Geometry: final body of the model. Coordinates: model frame, mm. Give positions to 0.01 mm unless a question says otherwise; leave off trailing zeros. Loops run counter-clockwise (first coordinate to the right, second up) from the corner with the lowest first, then second, coordinate; pieces in that order, holes last.
from build123d import *

# Parameters (mm, degrees)
F0_R           = 3.3999999346
F0_R_2         = 4.4999999135
F1_DEPTH       = 15
F2_D           = 8.8
F2_CBORE_D     = 15
F2_CBORE_DEPTH = 8
F3_D           = 8.8
F3_CBORE_D     = 15
F3_CBORE_DEPTH = 8.6
F4_D           = 8.8
F5_D           = 7.2


with BuildPart() as f1:
    # F0 (on Front) → F1 (new body)
    with BuildSketch(Plane.XZ):
        Polygon((25.9961503957, 121.2465122815), (-26.0038496043, 121.2465122815), (-34.0038514504, 113.2465114353), (-34.0038514504, -70.7534860262), (-26.0038496043, -78.7534868724), (25.9961503957, -78.7534868724), (33.9961512419, -70.7534860262), (33.9961512419, 113.2465114353), align=None)
        with Locations((-23.2538496572, -28.7534868339)):
            Circle(F0_R, mode=Mode.SUBTRACT)
        with Locations((-0.0038501043, -63.7534861608)):
            Circle(F0_R_2, mode=Mode.SUBTRACT)
        with Locations((23.2461494486, -28.7534868339)):
            Circle(F0_R, mode=Mode.SUBTRACT)
        with Locations((-23.2538496572, 71.246511243)):
            Circle(F0_R, mode=Mode.SUBTRACT)
        with Locations((23.2461494486, 71.246511243)):
            Circle(F0_R, mode=Mode.SUBTRACT)
        with Locations((-0.0038501043, 106.2465105699)):
            Circle(F0_R_2, mode=Mode.SUBTRACT)
    extrude(amount=F1_DEPTH)

    # F2 (through all)
    with Locations(Plane(origin=(0, 0, 0), x_dir=(1, 0, 0), z_dir=(0, 1, 0))):
        with Locations((-0.0038501043, -106.2465105699)):
            CounterBoreHole(F2_D / 2, F2_CBORE_D / 2, F2_CBORE_DEPTH)

    # F3 (through all)
    with Locations(Plane(origin=(0, 0, 0), x_dir=(1, 0, 0), z_dir=(0, 1, 0))):
        with Locations((-0.0038501043, 63.7534861608)):
            CounterBoreHole(F3_D / 2, F3_CBORE_D / 2, F3_CBORE_DEPTH)

    # F4 (through all)
    with Locations(Plane(origin=(0, 0, 0), x_dir=(1, 0, 0), z_dir=(0, 1, 0))):
        with Locations((23.2461494486, 28.7534868339)):
            Hole(F4_D / 2)

    # F5 (through all)
    with Locations(Plane(origin=(0, 0, 0), x_dir=(1, 0, 0), z_dir=(0, 1, 0))):
        with Locations((0, 0)):
            Hole(F5_D / 2)


solid = f1.part
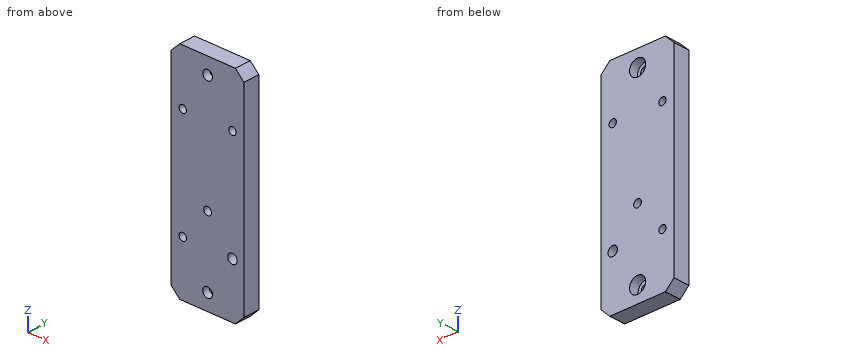
Item 1: Section query A-A on z = 0. Return loops of the section in (x, y), plus the area to 3 significant figures.
Values follow:
outline: (-34, -15) - (-3.6, -15) - (-3.6, 0) - (-34, 0) - close; (3.6, -15) - (34, -15) - (34, 0) - (3.6, 0) - close
area: 912 mm2
Item 2: Section query B-B on x = 0. Return loops of the section in (y, z).
Values follow:
outline: (-15, -78.75) - (0, -78.75) - (0, -71.25) - (-8.6, -71.25) - (-8.6, -68.25) - (-15, -68.25) - close; (-15, -59.25) - (-8.6, -59.25) - (-8.6, -56.25) - (0, -56.25) - (0, -3.6) - (-15, -3.6) - close; (-15, 3.6) - (0, 3.6) - (0, 98.75) - (-8, 98.75) - (-8, 101.75) - (-15, 101.75) - close; (-15, 110.75) - (-8, 110.75) - (-8, 113.75) - (0, 113.75) - (0, 121.25) - (-15, 121.25) - close
Item 3: Section query D-D on y = -4.25. Return loops of the section in (x, z).
Values follow:
outline: (-34, -70.75) - (-26, -78.75) - (26, -78.75) - (34, -70.75) - (34, 113.25) - (26, 121.25) - (-26, 121.25) - (-34, 113.25) - close; hole circle Ø6.8 at (-23.25, -28.75); hole circle Ø6.8 at (-23.25, 71.25); hole circle Ø15 at (0, -63.75); hole circle Ø15 at (0, 106.25); hole circle Ø7.2 at (0, 0); hole circle Ø8.8 at (23.25, -28.75); hole circle Ø6.8 at (23.25, 71.25)
Item 4: Ray query, probe 1 along Z at (x, y) = (0, -8.5); probe 2 along Z at (x, y) = (3, -4.5); probe 3 along Z at (x, y) = (22, -7.25). Return the intervals inside material, ascending.
Values follow:
probe 1: z = -78.75 to -71.25, -56.25 to -3.6, 3.6 to 101.75, 110.75 to 121.25
probe 2: z = -78.75 to -70.63, -56.88 to -1.99, 1.99 to 99.37, 113.12 to 121.25
probe 3: z = -78.75 to -32.97, -24.53 to 68.08, 74.41 to 121.25
Item 5: Section query C-C on y = -12.5. Return loops of the section in (x, z).
Values follow:
outline: (-34, -70.75) - (-26, -78.75) - (26, -78.75) - (34, -70.75) - (34, 113.25) - (26, 121.25) - (-26, 121.25) - (-34, 113.25) - close; hole circle Ø6.8 at (-23.25, -28.75); hole circle Ø6.8 at (-23.25, 71.25); hole circle Ø9 at (0, -63.75); hole circle Ø9 at (0, 106.25); hole circle Ø7.2 at (0, 0); hole circle Ø8.8 at (23.25, -28.75); hole circle Ø6.8 at (23.25, 71.25)
Item 6: Pin query (flat end, axial travel): pin 1 (8 mm diameter, centred on x = -3, z = 83.5, fed in from +Y); pin 2 (7.5 mm diameter, centred on x = -2.5, z = -63, fed in from +Y); pin 3 (1 mm diameter, centred on x = -27, y = -3, fed in from +Z); pin 4 (4.5 mm diameter, centred on x = 0, z = 0, fed in from +Y). Return the tip coordinate at first contact, or that it passes through.
Values follow:
pin 1: stops at y = 0
pin 2: stops at y = -8.6
pin 3: stops at z = 120.75
pin 4: passes through
